Input: part model. Units: mm. Frame: model coordinates. A direction names the side the tool comes from. Give positions to 0.01 mm unless a question says otherwise; leave off trailing zeros. Loops run counter-clockwise (first coordinate to the right, second up) from the corner with the lowest first, then second, coordinate; pieces in that order, holes last. Notation, with made-up numbers: M -16,17.25 L 40,17.25 A22 cw 40,53.25 Z; hole C 59,61 d9. An arc over 180 degrees is marked long. Use CSV: the item, a comma, the result in double quotes. Start each with the question number.
Q1. Section B-B, the plane y = 37.5. Output: boundary loops of the cut face in (x, z), plus the area to 3 significant figures.
Q2. Section A-A, the plane x = 110. Output: boundary loops of the cut face in (y, z).
Q3. Section C-C, the plane z = 84. Output: boundary loops of the cut face in (x, y).
Q4. Reachability of faces 1 (the flat face through (89, 30, 20)), 2 (the flat face through (185, 23.5, 10)), 3 (the flat face through (0, 37, 47)) from +Z, -Z, +X, -X, +Y, -Y: full face, straight path, thin tool, end or side. Return the list, or none.
Q5. Material intervals for line 1 along X through (y, z) = (32, 57.5); line 2 along Z through (x, y) = (215, 37); line 3 along Z through (x, y) = (108, 61), sorted ascending.
Q6. Pin query (flat end, axial travel): pin 1 (3 mm diameter, centred on x = 185, z = 8, fed in from -Y); pin 2 (6.5 mm diameter, centred on y = 37.5, z = 71, fed in from -X); pin 3 (4 mm diameter, centred on x = 58, y = 10.5, fed in from +Z). Return the tip coordinate at first contact, or that it passes through.
Q7. Section D-D, the plane y = 67.5. Output: boundary loops of the cut face in (x, z), plus the area to 3 significant figures.
Q8. Pull-direction query (Y, two-part tool) for faces 4 (the flat face through (108, 0, 15)), 5 (the flat face through (10, 38, 96)), 6 (the flat face through (153, 51.5, 10)); classes: released by +Y, released by -Y, zero draft, split by the parting line, or undercut.
from build123d import *

# Parameters (mm, degrees)
ESQUISSE1_W             = 220
ESQUISSE1_H             = 75
BOSS_EXTRU_1_DEPTH      = 20
ESQUISSE2_W             = 20
ESQUISSE2_H             = 75
BOSS_EXTRU_2_DEPTH      = 76
ESQUISSE3_R             = 4
ENL_V_MAT_EXTRU_1_DEPTH = 252.4776332
ESQUISSE4_R             = 22
ENL_V_MAT_EXTRU_2_DEPTH = 76
ESQUISSE5_R             = 1.5
ENL_V_MAT_EXTRU_3_DEPTH = 252.4776332
ENL_V_MAT_EXTRU_5_DEPTH = 245.542429856


with BuildPart() as part:
    # Esquisse1 → Boss.-Extru.1 (new body)
    with BuildSketch(Plane.XY):
        with Locations((110, 37.5)):
            Rectangle(ESQUISSE1_W, ESQUISSE1_H)
    extrude(amount=BOSS_EXTRU_1_DEPTH)

    # Esquisse2 → Boss.-Extru.2 (add)
    with BuildSketch(Plane.XY.offset(20)):
        with Locations((210, 37.5)):
            Rectangle(ESQUISSE2_W, ESQUISSE2_H)
        with Locations((10, 37.5)):
            Rectangle(ESQUISSE2_W, ESQUISSE2_H)
    extrude(amount=BOSS_EXTRU_2_DEPTH)

    # Esquisse3 → Enlèv. mat.-Extru.1 (cut, through all)
    with BuildSketch(Plane(origin=(220, 0, 0), x_dir=(0, 0, -1), z_dir=(1, 0, 0))):
        with Locations((-71, 37.5)):
            Circle(ESQUISSE3_R)
    extrude(amount=-ENL_V_MAT_EXTRU_1_DEPTH, mode=Mode.SUBTRACT)

    # Esquisse4 → Enlèv. mat.-Extru.2 (cut)
    with BuildSketch(Plane.XY.offset(20)):
        with Locations((110, 37.5)):
            Circle(ESQUISSE4_R)
    extrude(amount=-ENL_V_MAT_EXTRU_2_DEPTH, mode=Mode.SUBTRACT)

    # Esquisse5 → Enlèv. mat.-Extru.3 (cut, through all)
    with BuildSketch(Plane(origin=(220, 0, 0), x_dir=(0, 0, -1), z_dir=(1, 0, 0))):
        with Locations((-70.685514893, 47)):
            Circle(ESQUISSE5_R)
        with Locations((-62.61551611, 41.977647908)):
            Circle(ESQUISSE5_R)
        with Locations((-62.930001218, 32.477647908)):
            Circle(ESQUISSE5_R)
        with Locations((-71.314485107, 28)):
            Circle(ESQUISSE5_R)
        with Locations((-79.38448389, 33.022352092)):
            Circle(ESQUISSE5_R)
        with Locations((-79.069998782, 42.522352092)):
            Circle(ESQUISSE5_R)
    extrude(amount=-ENL_V_MAT_EXTRU_3_DEPTH, mode=Mode.SUBTRACT)

    # Esquisse6 → Enlèv. mat.-Extru.5 (cut, through all)
    with BuildSketch(Plane.XY.offset(20)):
        with BuildLine():
            Line((182.5, 54.5), (186.5, 54.5))
            ThreePointArc((186.5, 54.5), (188, 53), (186.5, 51.5))
            Line((186.5, 51.5), (182.5, 51.5))
            ThreePointArc((182.5, 51.5), (181, 53), (182.5, 54.5))
        make_face()
        with BuildLine():
            Line((151.5, 51.5), (155.5, 51.5))
            ThreePointArc((155.5, 51.5), (157, 53), (155.5, 54.5))
            Line((155.5, 54.5), (151.5, 54.5))
            ThreePointArc((151.5, 54.5), (150, 53), (151.5, 51.5))
        make_face()
        with BuildLine():
            Line((151.5, 20.5), (155.5, 20.5))
            ThreePointArc((155.5, 20.5), (157, 22), (155.5, 23.5))
            Line((155.5, 23.5), (151.5, 23.5))
            ThreePointArc((151.5, 23.5), (150, 22), (151.5, 20.5))
        make_face()
        with BuildLine():
            Line((182.5, 20.5), (186.5, 20.5))
            ThreePointArc((186.5, 20.5), (188, 22), (186.5, 23.5))
            Line((186.5, 23.5), (182.5, 23.5))
            ThreePointArc((182.5, 23.5), (181, 22), (182.5, 20.5))
        make_face()
    extrude(amount=-ENL_V_MAT_EXTRU_5_DEPTH, mode=Mode.SUBTRACT)


solid = part.part
A:
1,outline,"M 0,0 L 88,0 L 88,20 L 20,20 L 20,67 L 0,67 Z; M 0,75 L 20,75 L 20,96 L 0,96 Z; M 132,0 L 220,0 L 220,67 L 200,67 L 200,20 L 132,20 Z; M 200,75 L 220,75 L 220,96 L 200,96 Z"
1,area,"6,240 mm^2"
2,outline,"M 0,0 L 15.5,0 L 15.5,20 L 0,20 Z; M 59.5,0 L 75,0 L 75,20 L 59.5,20 Z"
3,outline,"M 0,0 L 20,0 L 20,75 L 0,75 Z; M 200,0 L 220,0 L 220,75 L 200,75 Z"
4,face 1,"+Z, +Y, -Y"
4,face 2,"+Z, -Z"
4,face 3,"+Z, -Z, -X, +Y, -Y"
5,line 1,"0 to 20, 200 to 220"
5,line 2,"0 to 67.03, 74.97 to 96"
5,line 3,"0 to 20"
6,pin 1,"y = 0"
6,pin 2,"through"
6,pin 3,"z = 20"
7,outline,"M 0,0 L 220,0 L 220,96 L 200,96 L 200,20 L 20,20 L 20,96 L 0,96 Z"
7,area,"7,440 mm^2"
8,face 4,"released by -Y"
8,face 5,"zero draft"
8,face 6,"undercut"
